Build history of the part. All positions in model axes, mm. A direction names the side the tool comes from. Round coordinates to 2 decimals unless told otherwise and drop trailing zeros. Order: outer loops, then holes, each group sorted by start corner. A loop starts at its lowest first (then second) coordinate and runs counter-clockwise, first axis right, second up. Notation, with made-up numbers: M 59,-15.5 L 85,-15.5 A13 ccw 85,7.5 Z; hole C 26,30.5 d11. An arc over 180 degrees is marked long. Use CSV: the item, a comma, the result in double quotes.
from build123d import *

# Parameters (mm, degrees)
F0_W     = 63.5
F0_H     = 76.2
F1_DEPTH = 3.175
F2_W     = 3.175
F2_H     = 12.7
F3_DEPTH = 3.176


# Not quite as in the source:
# - a pattern or mirror of a feature is missing from the dataset's text; its kind, count and spacing are read off the source's solid


with BuildPart() as f1:
    # F0 (on Front) → F1 (new body)
    with BuildSketch(Plane.XZ):
        Rectangle(F0_W, F0_H)
    extrude(amount=F1_DEPTH)

    # F2 (on Front) → F3 (cut, through all)
    with BuildSketch(Plane.XZ):
        with Locations((-30.1625, 19.05)):
            Rectangle(F2_W, F2_H)
        with Locations((-30.1625, -6.35)):
            Rectangle(F2_W, F2_H)
        with Locations((-30.1625, -31.75)):
            Rectangle(F2_W, F2_H)
    f3 = extrude(amount=F3_DEPTH, mode=Mode.SUBTRACT)

    # F3_copies: F3 across plane
    add(f3.mirror(Plane(origin=(0, 0, 0), x_dir=(0, 0, 1), z_dir=(1, 0, 0))), mode=Mode.SUBTRACT)


solid = f1.part
(1) Drop flat-ended pins along their axis: pin 1 (1.6 mm diameter, centred on y = -2, z = -33.5, fed in from -X) (3 decimals); pin 2 (1 mm diameter, centred on y = -2, z = -8.5, fed in from +X) (3 decimals); pin 3 (1 mm diameter, centred on x = 29.5, y = -2, fed in from -Z). Give the stop position or say it passes through.
Answer block:
pin 1,"stops at x = -28.575"
pin 2,"stops at x = 28.575"
pin 3,"stops at z = -25.4"
(2) Wall check: line 1 (Z direction, x = 29, y = -0.2); line 2 (X direction, y = -1.7, z = 24.5) (3 decimals). Give the ranges that are in metal, low to high. Write a range as from..to.
Answer block:
line 1,"z = -25.4..-12.7, 0..12.7, 25.4..38.1"
line 2,"x = -28.575..28.575"
(3) Tool access for faces 1 (the face through (30, -2, 25.4)), 2 (the face through (-28.575, -2, -32)), 3 (the face through (-30, -2, 0)): list every direction of +Z, -Z, +X, -X, +Y, -Y with a clear straight run to the whole face (end or side of a thin tool).
Answer block:
face 1,"+X, +Y, -Y"
face 2,"-Z, -X, +Y, -Y"
face 3,"-X, +Y, -Y"
(4) Cut at B-B, the plane z = -29. Give the cut face in (x, y) (3 decimals).
Answer block:
outline,"M -28.575,-3.175 L 28.575,-3.175 L 28.575,0 L -28.575,0 Z"
(5) Cut at A-A, the plane y = -2.15. Give the cut face in (x, z) (3 decimals).
Answer block:
outline,"M -31.75,-25.4 L -28.575,-25.4 L -28.575,-38.1 L 28.575,-38.1 L 28.575,-25.4 L 31.75,-25.4 L 31.75,-12.7 L 28.575,-12.7 L 28.575,0 L 31.75,0 L 31.75,12.7 L 28.575,12.7 L 28.575,25.4 L 31.75,25.4 L 31.75,38.1 L -31.75,38.1 L -31.75,25.4 L -28.575,25.4 L -28.575,12.7 L -31.75,12.7 L -31.75,0 L -28.575,0 L -28.575,-12.7 L -31.75,-12.7 Z"
(6) Two-plate mould, pull along Z, no slides. Class faces 4 (the face through (31.75, -2, -19)), 5 (the face through (0, -2, -38.1)), 6 (the face through (-30, -2, -12.7)): released by +Z, released by -Z, zero draft, split by the parting line, or undercut.
Answer block:
face 4,"zero draft"
face 5,"released by -Z"
face 6,"undercut"
